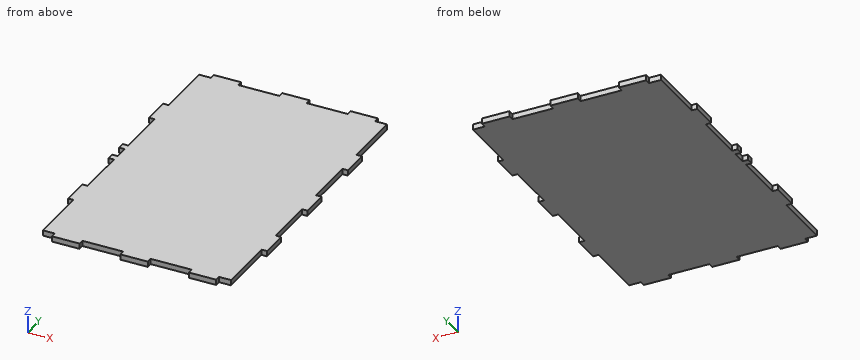
Autodesk Inventor part; units mm, degrees
ref_plane "YZ Plane" through (0, 0, 0) normal (1, 0, 0) x (0, 1, 0)
ref_plane "XZ Plane" through (0, 0, 0) normal (0, 1, 0) x (-1, 0, 0)
ref_plane "XY Plane" through (0, 0, 0) normal (0, 0, 1) x (1, 0, 0)
sketch "Sketch1" plane through (0, 0, 0) normal (0, 0, 1) x (1, 0, 0)
  line L0 (0, 62.09) -> (0, -62.09) construction
  line L1 (-38.5, 0) -> (38.5, 0) construction
  line L2 (27.5, -44.35) -> (-27.5, -44.35)
  line L3 (-27.5, -44.35) -> (-27.5, 44.35)
  line L4 (-27.5, 44.35) -> (27.5, 44.35)
  line L5 (27.5, 44.35) -> (27.5, -44.35)
  line L6 (27.5, -44.35) -> (-27.5, 44.35) construction
  line L7 (-27.5, -44.35) -> (27.5, 44.35) construction
  point P0 (0, 0)
  dimension "d0" = 55
  dimension "d1" = 88.7
extrude "Extrusion1" add sketch "Sketch1" along normal mid plane 1.6
sketch "Esquisse2" plane through (0, 0, 0.8) normal (0, 0, 1) x (1, 0, 0)
  line L0 (-27.5, -44.35) -> (27.5, -44.35) construction
  line L1 (27.5, -44.35) -> (27.5, 44.35) construction
  line L2 (27.5, 44.35) -> (-27.5, 44.35) construction
  line L3 (-27.5, 44.35) -> (-27.5, -44.35) construction
  line L4 (0, 62.09) -> (0, -62.09) construction
  line L5 (-40.42, 0) -> (38.82, 0) construction
  line L6 (-27.5, -27) -> (-29.1, -27)
  line L7 (-29.1, -27) -> (-29.1, -19)
  line L8 (-29.1, -19) -> (-27.5, -19)
  line L9 (-27.5, -19) -> (-27.5, -27)
  line L10 (-27.5, -4) -> (-29.1, -4)
  line L11 (-29.1, -4) -> (-29.1, 4)
  line L12 (-29.1, 4) -> (-27.5, 4)
  line L13 (-27.5, 4) -> (-27.5, -4)
  line L14 (-27.5, 19) -> (-29.1, 19)
  line L15 (-29.1, 19) -> (-29.1, 27)
  line L16 (-29.1, 27) -> (-27.5, 27)
  line L17 (-27.5, 27) -> (-27.5, 19)
  point P0 (0, 0)
  dimension "d4" = 1.6
  dimension "d5" = 8
  dimension "d8" = 23
extrude "Extrusion2" add sketch "Esquisse2" against normal blind 1.6
mirror "Symétrie1" about plane through (0, 0, 0) normal (1, 0, 0) of "Extrusion2"
sketch "Esquisse3" plane through (0, 0, 0.8) normal (0, 0, 1) x (1, 0, 0)
  line L0 (-29.1, 27) -> (-27.5, 27) construction
  line L1 (-27.5, 27) -> (-27.5, 44.35) construction
  line L2 (-27.5, 44.35) -> (27.5, 44.35) construction
  line L3 (27.5, 44.35) -> (27.5, 27) construction
  line L4 (27.5, 27) -> (29.1, 27) construction
  line L5 (29.1, 27) -> (29.1, 19) construction
  line L6 (29.1, 19) -> (27.5, 19) construction
  line L7 (27.5, 19) -> (27.5, 4) construction
  line L8 (27.5, 4) -> (29.1, 4) construction
  line L9 (29.1, 4) -> (29.1, -4) construction
  line L10 (29.1, -4) -> (27.5, -4) construction
  line L11 (27.5, -4) -> (27.5, -19) construction
  line L12 (27.5, -19) -> (29.1, -19) construction
  line L13 (29.1, -19) -> (29.1, -27) construction
  line L14 (29.1, -27) -> (27.5, -27) construction
  line L15 (27.5, -27) -> (27.5, -44.35) construction
  line L16 (27.5, -44.35) -> (-27.5, -44.35) construction
  line L17 (-27.5, -44.35) -> (-27.5, -27) construction
  line L18 (-27.5, -27) -> (-29.1, -27) construction
  line L19 (-29.1, -27) -> (-29.1, -19) construction
  line L20 (-29.1, -19) -> (-27.5, -19) construction
  line L21 (-27.5, -19) -> (-27.5, -4) construction
  line L22 (-27.5, -4) -> (-29.1, -4) construction
  line L23 (-29.1, -4) -> (-29.1, 4) construction
  line L24 (-29.1, 4) -> (-27.5, 4) construction
  line L25 (-27.5, 4) -> (-27.5, 19) construction
  line L26 (-27.5, 19) -> (-29.1, 19) construction
  line L27 (-29.1, 19) -> (-29.1, 27) construction
  line L28 (0, 62.09) -> (0, -62.09) construction
  line L29 (-40.74, 0) -> (40.74, 0) construction
  line L30 (-27.5, -44.35) -> (27.5, -44.35) construction
  line L31 (27.5, -44.35) -> (27.5, -27) construction
  line L32 (27.5, -27) -> (29.1, -27) construction
  line L33 (29.1, -27) -> (29.1, -19) construction
  line L34 (29.1, -19) -> (27.5, -19) construction
  line L35 (27.5, -19) -> (27.5, -4) construction
  line L36 (27.5, -4) -> (29.1, -4) construction
  line L37 (29.1, -4) -> (29.1, 4) construction
  line L38 (29.1, 4) -> (27.5, 4) construction
  line L39 (27.5, 4) -> (27.5, 19) construction
  line L40 (27.5, 19) -> (29.1, 19) construction
  line L41 (29.1, 19) -> (29.1, 27) construction
  line L42 (29.1, 27) -> (27.5, 27) construction
  line L43 (27.5, 27) -> (27.5, 44.35) construction
  line L44 (27.5, 44.35) -> (-27.5, 44.35) construction
  line L45 (-27.5, 44.35) -> (-27.5, 27) construction
  line L46 (-29.1, 27) -> (-27.5, 27) construction
  line L47 (-29.1, 19) -> (-29.1, 27) construction
  line L48 (-27.5, 19) -> (-29.1, 19) construction
  line L49 (-27.5, 19) -> (-27.5, 4) construction
  line L50 (-29.1, 4) -> (-27.5, 4) construction
  line L51 (-29.1, -4) -> (-29.1, 4) construction
  line L52 (-27.5, -4) -> (-29.1, -4) construction
  line L53 (-27.5, -4) -> (-27.5, -19) construction
  line L54 (-29.1, -19) -> (-27.5, -19) construction
  line L55 (-29.1, -27) -> (-29.1, -19) construction
  line L56 (-27.5, -27) -> (-29.1, -27) construction
  line L57 (-27.5, -27) -> (-27.5, -44.35) construction
  line L58 (24, 44.35) -> (16, 44.35)
  line L59 (16, 44.35) -> (16, 45.95)
  line L60 (16, 45.95) -> (24, 45.95)
  line L61 (24, 45.95) -> (24, 44.35)
  line L62 (4, 44.35) -> (-4, 44.35)
  line L63 (-4, 45.95) -> (4, 45.95)
  line L64 (4, 45.95) -> (4, 44.35)
  line L65 (-4, 44.35) -> (-4, 45.95)
  line L66 (-16, 44.35) -> (-24, 44.35)
  line L67 (-24, 45.95) -> (-16, 45.95)
  line L68 (-16, 45.95) -> (-16, 44.35)
  line L69 (-24, 44.35) -> (-24, 45.95)
  point P0 (0, 0)
  dimension "d15" = 8
  dimension "d16" = 1.6
  dimension "d19" = 20
extrude "Extrusion3" add sketch "Esquisse3" against normal blind 1.6
mirror "Symétrie2" about plane through (0, 0, 0) normal (0, 1, 0) of "Extrusion3"
sketch "Esquisse4" plane through (-29.1, -4, 0.8) normal (-1, 0, 0) x (0, 0, 1)
  point P0 (-0.8, 4)
sketch "Esquisse5" plane through (0, 0, 0.8) normal (0, 0, 1) x (1, 0, 0)
  line L0 (-27.5, 31) -> (-29.1, 31)
  line L1 (-29.1, 31) -> (-29.1, 2)
  line L2 (-29.1, 2) -> (-27.5, 2)
  line L3 (-27.5, 2) -> (-27.5, -2)
  line L4 (-27.5, -2) -> (-29.1, -2)
  line L5 (-29.1, -2) -> (-29.1, -31)
  line L6 (-29.1, -31) -> (-27.5, -31)
  line L7 (-27.5, -31) -> (-27.5, -39)
  line L8 (-27.5, -39) -> (-29.1, -39)
  line L9 (-29.1, -39) -> (-29.1, -44.35)
  line L10 (-29.1, -44.35) -> (-32.6, -44.35)
  line L11 (-32.6, -44.35) -> (-32.6, -45.95)
  line L12 (-32.6, -45.95) -> (-40.6, -45.95)
  line L13 (-40.6, -45.95) -> (-40.6, -44.35)
  line L14 (-40.6, -44.35) -> (-44.1, -44.35)
  line L15 (-44.1, -44.35) -> (-44.1, 44.35)
  line L16 (-44.1, 44.35) -> (-29.1, 44.35)
  line L17 (-29.1, 44.35) -> (-29.1, 39)
  line L18 (-29.1, 39) -> (-27.5, 39)
  line L19 (-27.5, 39) -> (-27.5, 31)
  point P0 (0, 0)
extrude "Extrusion4" cut sketch "Esquisse5" against normal blind 1.6
properties part number "BaseSupportBatterie1" material "PVC-U"
CAD build for the part. Positions are in the model's coordinates, mm. Coordinates: 2 decimals unless noted, no trailing zeros. Write each loop counter-clockwise with the first axis right and the second up, starting at its lowest first coordinate (ties: lowest second). Pieces come first, ordered by that corner, then holes.
(1) Cut at B-B, the plane x = 9. List the corners of the cut face in (y, z), and give its area (3 significant figures).
(2) Cut at A-A, the plane y = -8. List the corners of the cut face in (x, z).
(3) Flat gauge pins, fed straight in: pin 1 (0.8 mm diameter, centred on x = 28, z = -0.5, fed in from +Y); pin 2 (0.8 mm diameter, centred on y = 45, z = 0, fed in from -X); pin 3 (0.5 mm diameter, centred on x = -25.5, z = 0.5, fed in from -Y). Where does each tip first touch, or does it go through?
(4) Drill centre lines: probe 1 along Y at (x, z) = (-26, 0.2); probe 2 along X at (y, z) = (12, -0.3). Where is each one in solid material? Low to high.
Geometry says:
1. outline: (-44.35, -0.8) - (44.35, -0.8) - (44.35, 0.8) - (-44.35, 0.8) - close
1. area: 142 mm2
2. outline: (-27.5, -0.8) - (27.5, -0.8) - (27.5, 0.8) - (-27.5, 0.8) - close
3. pin 1: stops at y = 27
3. pin 2: stops at x = -24
3. pin 3: stops at y = -44.35
4. probe 1: y = -44.35 to 44.35
4. probe 2: x = -27.5 to 27.5
